Design review of the part shown in the three views and the two pictorial views. Dimensions are in mm from the part's minimum x, y and z. Round coordinates to 2 decimals unless told otherwise and drop trailing zeros. Order: outer loops, then holes, each group sorted by start corner. A loop starts at its lowest first (then second) coordinate and runs counter-clockwise, first axis right, second up. Notation, with made-up numbers: (58.25, -28) - (109.25, -28) arc R22 ccw to (109.25, 3) - close; hole circle Ø9 at (-10, 32.25). An arc over 180 degrees is marked (long way). Use CSV: the item, a comma, the result in double quotes.
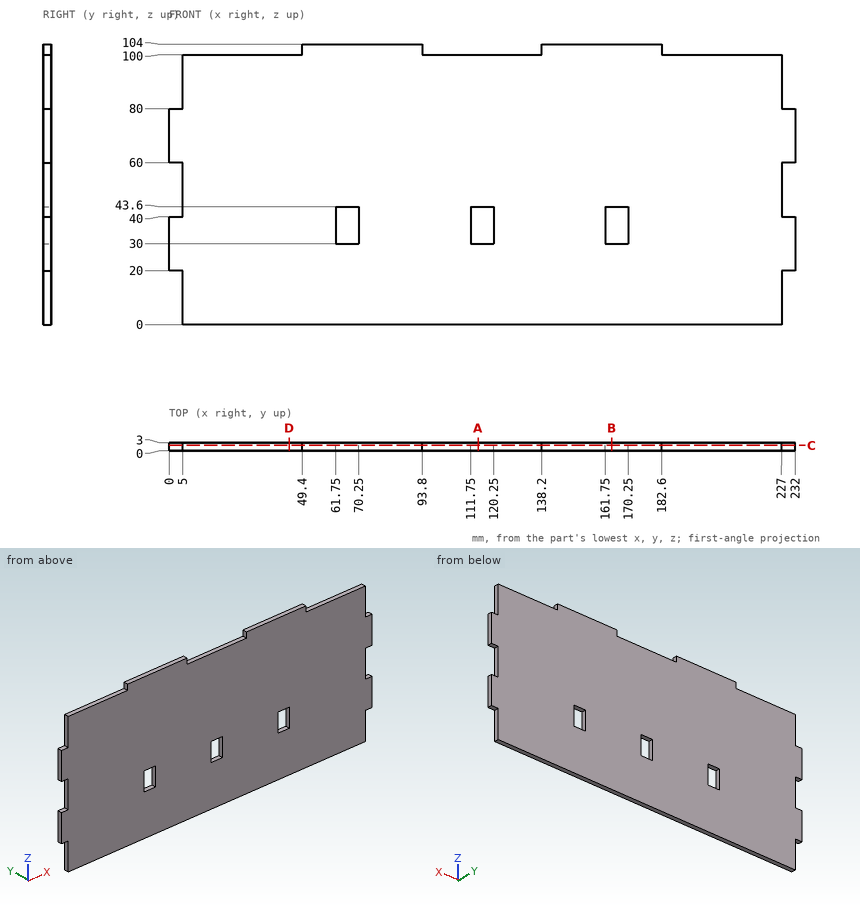
1) We need section C-C (y = 2). Give the number of separate pieces and of enclosed holes in the cut face, then the cut area to 3 significant figures.
Data:
separate pieces,"1"
enclosed holes,"3"
area,"22,600 mm2"
2) We need section B-B (x = 164). Give the boundary of the cut face in (y, z), then the cut area to 3 significant figures.
Data:
outline,"(0, 0) - (3, 0) - (3, 30) - (0, 30) - close; (0, 43.6) - (3, 43.6) - (3, 104) - (0, 104) - close"
area,"271 mm2"
3) We need section A-A (x = 114.5). Give the boundary of the cut face in (y, z).
Data:
outline,"(0, 0) - (3, 0) - (3, 30) - (0, 30) - close; (0, 43.6) - (3, 43.6) - (3, 100) - (0, 100) - close"
4) To check wall thickness, follow L1, parallel to X at y = 1.5, z = 40.5; L2, parallel to X at y = 1.35, z = 36.5; L3, parallel to Z at x = 67, y = 0.8. State the ranges of each line that lie inside material, in increasing order. Write a range as from..to.
Data:
L1,"x = 5..61.75, 70.25..111.75, 120.25..161.75, 170.25..227"
L2,"x = 0..61.75, 70.25..111.75, 120.25..161.75, 170.25..232"
L3,"z = 0..30, 43.6..104"
5) We need section D-D (x = 44.5). Give the boundary of the cut face in (y, z).
Data:
outline,"(0, 0) - (3, 0) - (3, 100) - (0, 100) - close"
6) Insertion check: pin 1 Ø0.9 at (y, z) = (1.5, 51.5) entering from +X; pin 2 Ø1.5 at (x, y) = (118, 1) entering from +Z; pin 3 Ø1.5 at (x, y) = (229, 1.5) entering from -Z. Each pin has a flat end and moves straight along its axis. Give the tip position at first contact, or say it passes through.
Data:
pin 1,"stops at x = 227"
pin 2,"stops at z = 100"
pin 3,"stops at z = 20"
